Source: CAD feature listing. Evaluate the final solid. Frame: model axes, mm. Face numbers are marked on the shaded views. A direction names the side the tool comes from. Round coordinates to 2 decimals unless told otherwise and drop trailing zeros. Loops run counter-clockwise (first coordinate to the right, second up) from the corner with the lowest first, then second, coordinate; pieces in that order, holes last. Notation, with made-up numbers: (37, 3.5) -> (96, 3.5) arc R15 cw to (96, 7.5) -> close; hole circle Ø5 at (-40, 33). An arc over 180 degrees is marked (long way). Write item = value, one per line.
from build123d import *

# Parameters (mm, degrees)
F0_W     = 76.2
F0_H     = 10.16
F1_DEPTH = 25.4
F0_W_2   = 5.584522
F0_H_2   = 101.6
F2_DEPTH = 25.4


with BuildPart() as f1:
    # F0 (on Top) → F1 (new body)
    with BuildSketch(Plane.XY):
        with Locations((5.793286, 36.60981)):
            Rectangle(F0_W, F0_H)
    extrude(amount=F1_DEPTH)

    # F0 (on Top) → F2 (join)
    with BuildSketch(Plane.XY):
        Polygon((-32.306714, -70.07019), (-32.306714, 31.52981), (-32.306714, 41.68981), (-39.255086, 41.68981), (-39.255086, -70.07019), align=None)
        with Locations((46.685547, -19.27019)):
            Rectangle(F0_W_2, F0_H_2)
        with Locations((46.685547, 36.60981)):
            Rectangle(F0_W_2, F0_H)
        with Locations((46.685547, -75.15019)):
            Rectangle(F0_W_2, F0_H)
        Polygon((43.893286, -80.23019), (43.893286, -70.07019), (-32.306714, -70.07019), (-39.255086, -70.07019), (-39.255086, -80.23019), align=None)
    extrude(amount=F2_DEPTH)


solid = f1.part
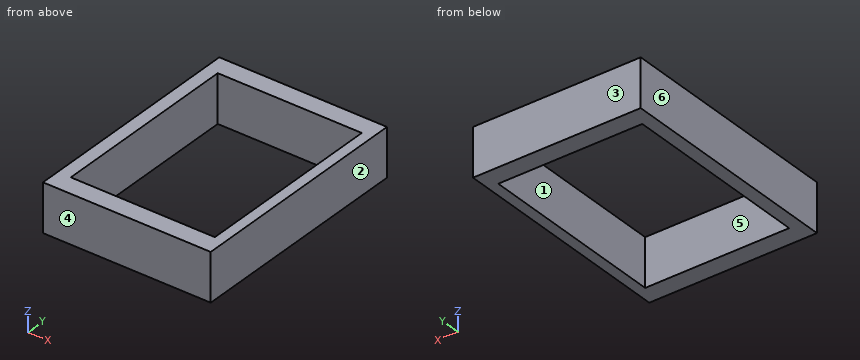
1. Section query A-A (y = 1.5). Return the cut outline in (x, z), then the cut area to 3 significant figures.
Evaluation:
outline = (-39.26, 0) -> (-32.31, 0) -> (-32.31, 25.4) -> (-39.26, 25.4) -> close; (43.89, 0) -> (49.48, 0) -> (49.48, 25.4) -> (43.89, 25.4) -> close
area = 318 mm²
2. Mould query, pull axis Y, two halves, no side actions, for the marked faces 3, 4, 5 and 6. Classes: released by +Y, released by -Y, zero draft, split by the parting line, or undercut.
Evaluation:
face_3 = released by +Y
face_4 = released by -Y
face_5 = undercut
face_6 = zero draft
3. Set-up query: the marked faces 1 and 2. Return all of +Z, -Z, +X, -X, +Y, -Y with unobstructed straight access to the full face (end or side cutting, diameter ignored); none if empty.
Evaluation:
face_1 = +Z, -Z
face_2 = +Z, -Z, +X, +Y, -Y
4. Section query C-C (z = 10.25). Return the cut outline in (x, y), then the cut area to 3 significant figures.
Evaluation:
outline = (-39.26, -80.23) -> (49.48, -80.23) -> (49.48, 41.69) -> (-39.26, 41.69) -> close; hole (-32.31, -70.07) -> (43.89, -70.07) -> (43.89, 31.53) -> (-32.31, 31.53) -> close
area = 3,080 mm²
5. Line query: probe 1 along Y at (x, z) = (17, 2.5); probe 2 along X at (y, z) = (13, 19.75). Output: solid intervals per line, ascending. Write a range as from..to.
Evaluation:
probe_1 = -80.23..-70.07, 31.53..41.69
probe_2 = -39.26..-32.31, 43.89..49.48
6. Section query B-B (x = 1). Return the cut outline in (y, z), then the cut area to 3 significant figures.
Evaluation:
outline = (-80.23, 0) -> (-70.07, 0) -> (-70.07, 25.4) -> (-80.23, 25.4) -> close; (31.53, 0) -> (41.69, 0) -> (41.69, 25.4) -> (31.53, 25.4) -> close
area = 516 mm²
